Geometry check sheet. Reference: the model listing, model coordinates, mm. A direction names the side the tool comes from. Coordinates: 2 decimals unless noted, no trailing zeros. Loops run counter-clockwise (first coordinate to the right, second up) from the corner with the lowest first, then second, coordinate; pieces in that order, holes last. Notation, with made-up numbers: (18, 47) - (67, 47) arc R11 cw to (67, 58) - close; hole circle Ø2 at (79.25, 58). An arc over 180 degrees is marked (long way). Write each question's results on one line, items separated by ' | '. Start each with the question number.
(1) Sectioned sample at D-D (x = 22.75). Enter the section's corners in (y, z).
(2) Mould release check, pull along Y, two halves, no side actions. Record for faces 3 (the face through (24.337, -1.638, 2.983)), 4 (the face through (0, 3, 4)), 5 (the face through (-15.413, -6.437, 3.944)), 6 (the face through (-26.03, -12.12, 3.94)): pulls with the +Y half, pulls with the -Y half, needs draft (parallel to the pull), parting line crosses it, or undercut.
(3) Access from +Z, -Z, +X, -X, +Y, -Y to the whole of each face (thin tool, end or side, straight path). Record for faces 1 (the face through (-17.5, 6, 4)), 2 (the face through (-28, 0, 4)).
(4) Sectioned sample at B-B (y = -5.22). Enter the section's corners in (x, z), plus the area to 3 significant figures.
(5) Material ranges on probe 1 along X at (y, z) = (-5.22, 5); probe 2 along X at (y, z) = (-0.25, 4); probe 3 along Y at (x, z) = (17, 5.5), recorded low to high.
(6) Sectioned sample at C-C (z = 3). Enter the section's corners in (x, y), plus the area to 3 significant figures.
(7) Sectioned sample at A-A (x = 17). Enter the section's corners in (y, z).
(8) Go/stop test with flat-tipped pins: pin 1 Ø3 at (x, y) = (-17, -5.22) entering from -Z; pin 2 Ø4 at (x, z) = (-1.5, 2.5) entering from +Y; pin 3 Ø4.5 at (x, y) = (-22.75, -0.42) entering from +Z; pin 4 Ø12 at (x, y) = (4, 4.5) entering from +Z. Record where each tip stops, or that it passes through.
from build123d import *

# Parameters (mm, degrees)
BOSS_EXTRUDE1_DEPTH           = 8
CSK_FOR_M4_SFHCS1_D           = 4
CSK_FOR_M4_SFHCS1_DEPTH       = 13
CSK_FOR_M4_SFHCS1_CSINK_D     = 7.9
CSK_FOR_M4_SFHCS1_CSINK_ANGLE = 90
CSK_FOR_M4_SFHCS1_TIP         = 1.201721238
CSK_FOR_M4_SFHCS2_D           = 4
CSK_FOR_M4_SFHCS2_DEPTH       = 16
CSK_FOR_M4_SFHCS2_CSINK_D     = 7.9
CSK_FOR_M4_SFHCS2_CSINK_ANGLE = 90
CSK_FOR_M4_SFHCS2_TIP         = 1.201721238


with BuildPart() as part:
    # Sketch1 → Boss-Extrude1 (new body)
    with BuildSketch(Plane.XY):
        Polygon((28, 0), (28, 10), (17.5, 10), (17.5, 3), (-17.5, 3), (-17.5, 10), (-28, 10), (-28, 0), (-28, -10.842369627), (-24, -13.44), (24, -13.44), (28, -10.842369627), align=None)
    extrude(amount=BOSS_EXTRUDE1_DEPTH)

    # CSK for M4 SFHCS1
    with Locations(Plane(origin=(-695.683007616, 1385.247292614, 13), x_dir=(1, 0, 0), z_dir=(0, 0, 1))):
        with Locations((678.683007616, -1390.467292614), (712.683007616, -1390.467292614)):
            CounterSinkHole(CSK_FOR_M4_SFHCS1_D / 2, CSK_FOR_M4_SFHCS1_CSINK_D / 2, depth=CSK_FOR_M4_SFHCS1_DEPTH, counter_sink_angle=CSK_FOR_M4_SFHCS1_CSINK_ANGLE)
            with Locations((0, 0, -(CSK_FOR_M4_SFHCS1_DEPTH + CSK_FOR_M4_SFHCS1_TIP / 2))):  # 118° drill point
                Cone(0, CSK_FOR_M4_SFHCS1_D / 2, CSK_FOR_M4_SFHCS1_TIP, mode=Mode.SUBTRACT)

    # CSK for M4 SFHCS2
    with Locations(Plane(origin=(-695.683007616, 1385.247292614, 8), x_dir=(1, 0, 0), z_dir=(0, 0, 1))):
        with Locations((672.933007616, -1385.668477427), (718.433007616, -1385.668477427)):
            CounterSinkHole(CSK_FOR_M4_SFHCS2_D / 2, CSK_FOR_M4_SFHCS2_CSINK_D / 2, depth=CSK_FOR_M4_SFHCS2_DEPTH, counter_sink_angle=CSK_FOR_M4_SFHCS2_CSINK_ANGLE)
            with Locations((0, 0, -(CSK_FOR_M4_SFHCS2_DEPTH + CSK_FOR_M4_SFHCS2_TIP / 2))):  # 118° drill point
                Cone(0, CSK_FOR_M4_SFHCS2_D / 2, CSK_FOR_M4_SFHCS2_TIP, mode=Mode.SUBTRACT)


solid = part.part
Outcome:
1) outline: (-13.44, 0) - (-2.42, 0) - (-2.42, 6.05) - (-4.37, 8) - (-13.44, 8) - close; (1.58, 0) - (10, 0) - (10, 8) - (3.53, 8) - (1.58, 6.05) - close
2) face 3: undercut | face 4: pulls with the +Y half | face 5: undercut | face 6: pulls with the -Y half
3) face 1: +Z, -Z, +Y | face 2: +Z, -Z, -X, +Y, -Y
4) outline: (-28, 0) - (-19, 0) - (-19, 8) - (-28, 8) - close; (-15, 0) - (15, 0) - (15, 8) - (-15, 8) - close; (19, 0) - (28, 0) - (28, 8) - (19, 8) - close | area: 384 mm2
5) probe 1: x = -28 to -19, -15 to 15, 19 to 28 | probe 2: x = -28 to -24.74, -20.76 to 20.76, 24.74 to 28 | probe 3: y = -13.44 to -7.22, -3.22 to 3
6) outline: (-28, -10.84) - (-24, -13.44) - (24, -13.44) - (28, -10.84) - (28, 10) - (17.5, 10) - (17.5, 3) - (-17.5, 3) - (-17.5, 10) - (-28, 10) - close; hole circle Ø4 at (-22.75, -0.42); hole circle Ø4 at (-17, -5.22); hole circle Ø4 at (17, -5.22); hole circle Ø4 at (22.75, -0.42) | area: 1,010 mm2
7) outline: (-13.44, 0) - (-7.22, 0) - (-7.22, 8) - (-13.44, 8) - close; (-3.22, 0) - (3, 0) - (3, 8) - (-3.22, 8) - close
8) pin 1: passes through | pin 2: stops at y = 3 | pin 3: stops at z = 6.3 | pin 4: stops at z = 8
